Can you work these out from the model? Positions are in its coordinate system, mm. Give positions to 0.01 mm unless a question says otherwise; leave off trailing zeros. Order: outer loops, then holes, each group sorted by start corner. A loop starts at its lowest first (then second) coordinate and runs counter-clockwise, first axis right, second up.
Item 1: I want a section at A-A, the plane y = 0. Write out the boundary of the cut face in (x, z).
Item 2: If I drill on line 1 along X through (y, z) = (322, 1.5); line 2 along Y through (x, z) = (-176.5, 6); line 3 along X through (y, z) = (-208, 3.5), over which ranges is the centre line in solid material (lowest first)?
Item 3: I'm going to push flat-ended pins straight in: pin 1 Ø5.5 at (x, y) = (60.67, 324.58) entering from +Z; pin 2 Ø10 at (x, y) = (-60.67, 324.58) entering from -Z; pin 3 Ø1 at (x, z) = (183, 3) entering from +Y; pin 4 Ø1.5 at (y, z) = (-127, 1.5) entering from -X. Where does each tip first touch, or does it pass through?
Item 4: If we mould it in two halves opening along X, with no side actions, what happens to faces 1 (the cylindrical face through (-13.42, 304.504, 3.131)), 2 (the cylindrical face through (339.18, -106.81, 3.13)), 3 (the flat face through (-107, -288, 0))? For each: +X half, -X half, draft (parallel to the pull), parting line (faces both ways), or undercut.
Item 5: I want a section at B-B, the plane x = -93. Write out the boundary of the cut face in (y, z).
Item 6: I want a section at C-C, the plane z = 4.75. Count the separate pieces of the cut face and the enclosed holes in it, then the cut area to 3 significant figures.
Autodesk Inventor part; units mm, degrees
ref_plane "YZ Plane" through (0, 0, 0) normal (1, 0, 0) x (0, 1, 0)
ref_plane "XZ Plane" through (0, 0, 0) normal (0, 1, 0) x (-1, 0, 0)
ref_plane "XY Plane" through (0, 0, 0) normal (0, 0, 1) x (1, 0, 0)
sketch "Sketch1" plane through (0, 0, 0) normal (0, 0, 1) x (1, 0, 0)
  circle A0 centre (0, 0) radius 355.6
  circle A1 centre (0, 0) radius 304.8
  circle A2 centre (0, 330.2) radius 3.175
  circle A3 centre (0, 349.25) radius 3.175
  circle A4 centre (119.282, 307.9023) radius 3.175
  circle A5 centre (126.1637, 325.6659) radius 3.175
  circle A6 centre (222.4543, 244.0207) radius 3.175
  circle A7 centre (235.2882, 258.0989) radius 3.175
  circle A8 centre (295.5829, 147.1828) radius 3.175
  circle A9 centre (312.6358, 155.6741) radius 3.175
  circle A10 centre (328.7914, 30.467) radius 3.175
  circle A11 centre (347.7602, 32.2247) radius 3.175
  circle A12 centre (317.5948, -90.3635) radius 3.175
  circle A13 centre (335.9176, -95.5768) radius 3.175
  circle A14 centre (263.5053, -198.99) radius 3.175
  circle A15 centre (278.7075, -210.4701) radius 3.175
  circle A16 centre (173.8279, -280.7417) radius 3.175
  circle A17 centre (183.8564, -296.9383) radius 3.175
  circle A18 centre (60.6741, -324.5777) radius 3.175
  circle A19 centre (64.1745, -343.3034) radius 3.175
  circle A20 centre (-60.6741, -324.5777) radius 3.175
  circle A21 centre (-64.1745, -343.3034) radius 3.175
  circle A22 centre (-173.8279, -280.7417) radius 3.175
  circle A23 centre (-183.8564, -296.9383) radius 3.175
  circle A24 centre (-263.5053, -198.99) radius 3.175
  circle A25 centre (-278.7075, -210.4701) radius 3.175
  circle A26 centre (-317.5948, -90.3635) radius 3.175
  circle A27 centre (-335.9176, -95.5768) radius 3.175
  circle A28 centre (-328.7914, 30.467) radius 3.175
  circle A29 centre (-347.7602, 32.2247) radius 3.175
  circle A30 centre (-295.5829, 147.1828) radius 3.175
  circle A31 centre (-312.6358, 155.6741) radius 3.175
  circle A32 centre (-222.4543, 244.0207) radius 3.175
  circle A33 centre (-235.2882, 258.0989) radius 3.175
  circle A34 centre (-119.282, 307.9023) radius 3.175
  circle A35 centre (-126.1637, 325.6659) radius 3.175
  circle A36 centre (0, -330.2) radius 3.175
  line L0 (0, -308.356) -> (3.302, -308.356)
  line L1 (0, -308.356) -> (-3.175, -308.356)
  line L2 (3.302, -308.356) -> (3.302, -304.7821)
  line L3 (-3.175, -308.356) -> (-3.175, -304.7835)
  circle A37 centre (119.282, -307.9023) radius 3.175
  line L4 (111.391, -287.5334) -> (114.4701, -286.3406)
  line L5 (111.391, -287.5334) -> (108.4304, -288.6803)
  line L6 (114.4701, -286.3406) -> (113.179, -283.008)
  line L7 (108.4304, -288.6803) -> (107.1399, -285.3491)
  circle A38 centre (222.4543, -244.0207) radius 3.175
  line L8 (207.7381, -227.8778) -> (210.1783, -225.6533)
  line L9 (207.7381, -227.8778) -> (205.3917, -230.0168)
  line L10 (210.1783, -225.6533) -> (207.7706, -223.0122)
  line L11 (205.3917, -230.0168) -> (202.9849, -227.3767)
  circle A39 centre (295.5829, -147.1828) radius 3.175
  line L12 (276.029, -137.4461) -> (277.5008, -134.4903)
  line L13 (276.029, -137.4461) -> (274.6138, -140.2882)
  line L14 (277.5008, -134.4903) -> (274.3016, -132.8972)
  line L15 (274.6138, -140.2882) -> (271.4157, -138.6958)
  circle A40 centre (328.7914, -30.467) radius 3.175
  line L16 (307.0406, -28.4515) -> (307.3453, -25.1636)
  line L17 (307.0406, -28.4515) -> (306.7477, -31.613)
  line L18 (307.3453, -25.1636) -> (303.7866, -24.8338)
  line L19 (306.7477, -31.613) -> (303.1904, -31.2833)
  circle A41 centre (317.5948, 90.3635) radius 3.175
  line L20 (296.5847, 84.3856) -> (295.6811, 87.5616)
  line L21 (296.5847, 84.3856) -> (297.4536, 81.3318)
  line L22 (295.6811, 87.5616) -> (292.2436, 86.5835)
  line L23 (297.4536, 81.3318) -> (294.0174, 80.3542)
  circle A42 centre (263.5053, 198.99) radius 3.175
  line L24 (246.0734, 185.826) -> (244.0835, 188.4611)
  line L25 (246.0734, 185.826) -> (247.9868, 183.2923)
  line L26 (244.0835, 188.4611) -> (241.2315, 186.3073)
  line L27 (247.9868, 183.2923) -> (245.1358, 181.1394)
  circle A43 centre (173.8279, 280.7417) radius 3.175
  line L28 (162.3285, 262.1696) -> (159.5211, 263.9078)
  line L29 (162.3285, 262.1696) -> (165.028, 260.4981)
  line L30 (159.5211, 263.9078) -> (157.6397, 260.8693)
  line L31 (165.028, 260.4981) -> (163.1473, 257.4607)
  circle A44 centre (60.6741, 324.5777) radius 3.175
  line L32 (56.6603, 303.1057) -> (53.4145, 303.7124)
  line L33 (56.6603, 303.1057) -> (59.7812, 302.5222)
  line L34 (53.4145, 303.7124) -> (52.7578, 300.1994)
  line L35 (59.7812, 302.5222) -> (59.1248, 299.0105)
  circle A45 centre (-60.6741, 324.5777) radius 3.175
  line L36 (-56.6603, 303.1057) -> (-59.906, 302.4989)
  line L37 (-56.6603, 303.1057) -> (-53.5393, 303.6891)
  line L38 (-59.906, 302.4989) -> (-59.2493, 298.9859)
  line L39 (-53.5393, 303.6891) -> (-52.8829, 300.1774)
  circle A46 centre (-173.8279, 280.7417) radius 3.175
  line L40 (-162.3285, 262.1696) -> (-165.1359, 260.4313)
  line L41 (-162.3285, 262.1696) -> (-159.6291, 263.841)
  line L42 (-165.1359, 260.4313) -> (-163.2545, 257.3927)
  line L43 (-159.6291, 263.841) -> (-157.7484, 260.8035)
  circle A47 centre (-263.5053, 198.99) radius 3.175
  line L44 (-246.0734, 185.826) -> (-248.0633, 183.191)
  line L45 (-246.0734, 185.826) -> (-244.16, 188.3597)
  line L46 (-248.0633, 183.191) -> (-245.2113, 181.0372)
  line L47 (-244.16, 188.3597) -> (-241.3091, 186.2068)
  circle A48 centre (-317.5948, 90.3635) radius 3.175
  line L48 (-296.5847, 84.3856) -> (-297.4883, 81.2097)
  line L49 (-296.5847, 84.3856) -> (-295.7158, 87.4394)
  line L50 (-297.4883, 81.2097) -> (-294.0509, 80.2316)
  line L51 (-295.7158, 87.4394) -> (-292.2797, 86.4618)
  circle A49 centre (-328.7914, -30.467) radius 3.175
  line L52 (-307.0406, -28.4515) -> (-306.7359, -31.7394)
  line L53 (-307.0406, -28.4515) -> (-307.3336, -25.29)
  line L54 (-306.7359, -31.7394) -> (-303.1773, -31.4097)
  line L55 (-307.3336, -25.29) -> (-303.7763, -24.9604)
  circle A50 centre (-295.5829, -147.1828) radius 3.175
  line L56 (-276.029, -137.4461) -> (-274.5571, -140.4019)
  line L57 (-276.029, -137.4461) -> (-277.4442, -134.604)
  line L58 (-274.5571, -140.4019) -> (-271.3579, -138.8089)
  line L59 (-277.4442, -134.604) -> (-274.2462, -133.0115)
  circle A51 centre (-222.4543, -244.0207) radius 3.175
  line L60 (-207.7381, -227.8778) -> (-205.2979, -230.1024)
  line L61 (-207.7381, -227.8778) -> (-210.0844, -225.7389)
  line L62 (-205.2979, -230.1024) -> (-202.8902, -227.4612)
  line L63 (-210.0844, -225.7389) -> (-207.6776, -223.0987)
  circle A52 centre (-119.282, -307.9023) radius 3.175
  line L64 (-111.391, -287.5334) -> (-108.312, -288.7262)
  line L65 (-111.391, -287.5334) -> (-114.3516, -286.3865)
  line L66 (-108.312, -288.7262) -> (-107.021, -285.3937)
  line L67 (-114.3516, -286.3865) -> (-113.0611, -283.0552)
  line L68 (0, -342.9) -> (12.7, -342.9)
  line L69 (12.7, -342.9) -> (12.7, -349.25)
  line L70 (12.7, -349.25) -> (-12.7, -349.25)
  line L71 (-12.7, -349.25) -> (-12.7, -342.9)
  line L72 (-12.7, -342.9) -> (0, -342.9)
  line L73 (-63.0181, 337.0595) -> (-75.5018, 334.7255)
  line L74 (-75.5018, 334.7255) -> (-76.6688, 340.9674)
  line L75 (-76.6688, 340.9674) -> (-51.7014, 345.6354)
  line L76 (-51.7014, 345.6354) -> (-50.5344, 339.3935)
  line L77 (-50.5344, 339.3935) -> (-63.0181, 337.0595)
  circle A53 centre (0, 0) radius 304.8
  dimension "d1" = 711.2
  dimension "d3" = 609.6
  dimension "d6" = 6.35
  dimension "d7" = 6.35
  dimension "d10" = 360
  dimension "d13" = 6.35
  dimension "d15" = 3.302
  dimension "d18" = 360
  dimension "d20" = 342.9
  dimension "d21" = 12.7
  dimension "d22" = 6.35
  dimension "d23" = 25.4
  dimension "d26" = 360
extrude "Extrusion1" add sketch "Sketch1" along normal blind 6.35 contours A0 | A1 L22 L20 L21 L23 | L18 L16 L17 L19 A1 | A1 L26 L24 L25 L27 | L14 L12 L13 L15 A1 | A1 L30 L28 L29 L31 | L10 L8 L9 L11 A1 | A1 L34 L32 L33 L35 | L6 L4 L5 L7 A1 | A1 L38 L36 L37 L39 | A1 L42 L40 L41 L43 | L66 L64 L65 L67 A1 | A1 L46 L44 L45 L47 | L62 L60 L61 L63 A1 | A1 L50 L48 L49 L51 | L58 L56 L57 L59 A1 | A1 L54 L52 L53 L55
properties part number "laser circle 3D"
Results list:
1. outline: (-355.6, 0) - (-304.8, 0) - (-304.8, 6.35) - (-355.6, 6.35) - close; (304.8, 0) - (355.6, 0) - (355.6, 6.35) - (304.8, 6.35) - close
2. line 1: x = -150.89 to -62.53, -58.82 to 58.82, 62.53 to 150.89
2. line 2: y = -308.71 to -282.46, -279.03 to -248.5, 248.5 to 279.03, 282.46 to 308.71
2. line 3: x = -288.42 to -280.7, -276.71 to -222.8, 222.8 to 276.71, 280.7 to 288.42
3. pin 1: passes through
3. pin 2: stops at z = 0
3. pin 3: stops at y = 305.2
3. pin 4: stops at x = -332.43
4. face 1: undercut
4. face 2: parting line
4. face 3: draft
5. outline: (-343.22, 0) - (-290.27, 0) - (-290.27, 6.35) - (-343.22, 6.35) - close; (290.27, 0) - (343.22, 0) - (343.22, 6.35) - (290.27, 6.35) - close
6. separate pieces: 1
6. enclosed holes: 54
6. area: 103,000 mm2
